```python
from build123d import *

# Parameters (mm, degrees)
CROQUIS1_W              = 51.2
CROQUIS1_H              = 13.75
SALIENTE_EXTRUIR1_DEPTH = 1
SALIENTE_EXTRUIR2_DEPTH = 13.75
SALIENTE_EXTRUIR3_REACH = 82.173
CROQUIS4_W              = 13.75
CROQUIS4_H              = 1


with BuildPart() as part:
    # Croquis1 → Saliente-Extruir1 (new body)
    with BuildSketch(Plane(origin=(0, 0, 0), x_dir=(1, 0, 0), z_dir=(0, 1, 0))):
        with Locations((0, 6.875)):
            Rectangle(CROQUIS1_W, CROQUIS1_H)
    extrude(amount=SALIENTE_EXTRUIR1_DEPTH)

    # Croquis2 → Saliente-Extruir2 (add)
    with BuildSketch(Plane.XY):
        with BuildLine():
            Line((25.6, 36.08), (25.6, 37.08))
            ThreePointArc((25.6, 37.08), (44.14, 18.54), (25.6, 0))
            Line((25.6, 0), (25.6, 1))
            ThreePointArc((25.6, 1), (43.14, 18.54), (25.6, 36.08))
        make_face()
        with BuildLine():
            ThreePointArc((-25.6, 36.08), (-43.14, 18.54), (-25.6, 1))
            Line((-25.6, 1), (-25.6, 0))
            ThreePointArc((-25.6, 0), (-44.14, 18.54), (-25.6, 37.08))
            Line((-25.6, 37.08), (-25.6, 36.08))
        make_face()
    extrude(amount=-SALIENTE_EXTRUIR2_DEPTH)

    # Saliente-Extruir3: up to this face of the body (flat: up to its plane)
    saliente_extruir3_end = Plane(part.part.faces().sort_by_distance((25.6, 36.58, -6.875))[0])
    # Croquis4 → Saliente-Extruir3 (add, up to the picked face)
    with BuildSketch(Plane(origin=(-25.6, 0, 0), x_dir=(0, 0, -1), z_dir=(1, 0, 0)), mode=Mode.PRIVATE) as saliente_extruir3_sk1:
        with Locations((6.875, 36.58)):
            Rectangle(CROQUIS4_W, CROQUIS4_H)
    saliente_extruir3_tool1 = split(extrude(saliente_extruir3_sk1.sketch, amount=SALIENTE_EXTRUIR3_REACH, mode=Mode.PRIVATE), bisect_by=saliente_extruir3_end, keep=Keep.BOTH, mode=Mode.PRIVATE)
    add(saliente_extruir3_tool1.solids().sort_by(Axis((-25.6, 36.58, -6.875), (1, 0, 0)))[0])


solid = part.part
```
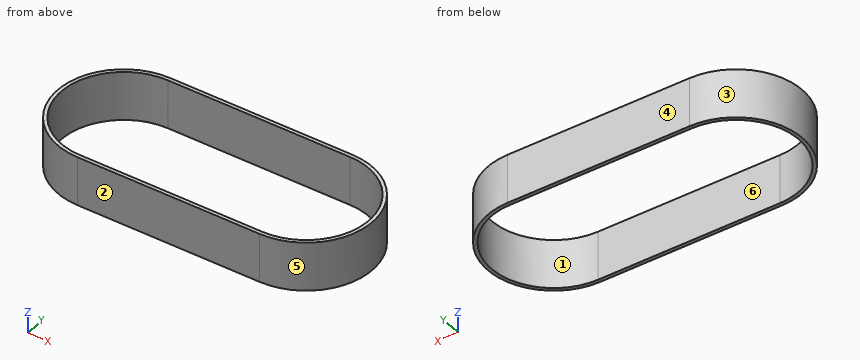
Can you work these out from the model? Positions are in its coordinate system, mm. Face numbers are marked on the shaded views. A direction names the side the tool comes from. Coordinates: 2 decimals unless noted, no trailing zeros. Order: outer loops, then holes, each group sorted by start corner. A loop starts at its lowest first (then second) coordinate and runs counter-clockwise, first axis right, second up. Notation, with made-up numbers: (24, 82.25) -> (75, 82.25) arc R15 ccw to (75, 89.25) -> close; hole circle Ø7 at (9.25, -11.75). An arc over 180 degrees is marked (long way). Write each question's results on one line, items separated by ' | '.
Item 1: I want a section at B-B, the plane x = 6.5. Write out the boundary of the cut face in (y, z), then the cut area to 3 significant figures.
Results are:
outline: (0, -13.75) -> (1, -13.75) -> (1, 0) -> (0, 0) -> close; (36.08, -13.75) -> (37.08, -13.75) -> (37.08, 0) -> (36.08, 0) -> close | area: 27.5 mm²
Item 2: I want a section at C-C, the plane z = -6. Write out the boundary of the cut face in (x, y).
Results are:
outline: (-25.6, 0) -> (25.6, 0) arc R18.54 ccw to (25.6, 37.08) -> (-25.6, 37.08) arc R18.54 ccw to start; hole (-25.6, 1) -> (25.6, 1) arc R17.54 ccw to (25.6, 36.08) -> (-25.6, 36.08) arc R17.54 ccw to start
Item 3: Which directions (+Z, -Z, +X, -X, +Y, -Y) give clear straight access to the entire face, cutting with the end or side of a thin tool? Please do the marked faces 5 and 6.
Results are:
face 5: +Z, -Z, +X | face 6: +Z, -Z
Item 4: If I drill on line 1 along Y through (x, z) = (23.5, -3); line 2 along X through (y, z) = (19.5, -6); line 3 along Y through (x, z) = (-32, -10), over which ranges is the centre line in solid material (lowest first)?
Results are:
line 1: 0 to 1, 36.08 to 37.08 | line 2: -44.12 to -43.11, 43.11 to 44.12 | line 3: 1.14 to 2.21, 34.87 to 35.94
Item 5: I want a section at A-A, the plane y = 18.54. Write out the boundary of the cut face in (x, z).
Results are:
outline: (-44.14, -13.75) -> (-43.14, -13.75) -> (-43.14, 0) -> (-44.14, 0) -> close; (43.14, -13.75) -> (44.14, -13.75) -> (44.14, 0) -> (43.14, 0) -> close
Item 6: If we mould it in two halves opening along Y, with no side actions, what happens to the marked faces 1, 2, 3 and 4? For each: +Y half, -Y half, draft (parallel to the pull), parting line (faces both ways), or undercut.
Results are:
face 1: undercut | face 2: -Y half | face 3: parting line | face 4: +Y half
Item 7: I'm going to push flat-ended pins straight in: pin 1 Ø1 at (y, z) = (10.5, -7) entering from +X; pin 2 Ø3 at (x, z) = (-28, -3) entering from +Y; pin 3 Ø2 at (x, z) = (32.5, -1.5) entering from +Y. Where does each tip first touch, or does it pass through?
Results are:
pin 1: x = 42.54 | pin 2: y = 37.06 | pin 3: y = 36.12
